```python
from build123d import *

# Parameters (mm, degrees)
F0_W     = 60
F0_H     = 40
F1_DEPTH = 70
F2_R     = 7.749318
F3_DEPTH = 15
F4_R     = 12.316216
F5_DEPTH = 15
F6_W     = 4.257482
F6_H     = 2.289564
F7_DEPTH = 5


with BuildPart() as f1:
    # F0 (on Top) → F1 (new body)
    with BuildSketch(Plane.XY):
        with Locations((-16.059712, 9.84915)):
            Rectangle(F0_W, F0_H)
    extrude(amount=F1_DEPTH)

    # F2 (on face) → F3 (join)
    with BuildSketch(Plane.XY.offset(70)):
        with Locations((-16.059712, 9.84915)):
            Circle(F2_R)
    extrude(amount=F3_DEPTH)

    # F4 (on face) → F5 (join)
    with BuildSketch(Plane.XY.offset(85)):
        with Locations((-16.059712, 9.84915)):
            Circle(F4_R)
    extrude(amount=F5_DEPTH)

    # F6 (on face) → F7 (join)
    with BuildSketch(Plane.XY.offset(100)):
        with Locations((-13.930971, 8.704368)):
            Rectangle(F6_W, F6_H)
    extrude(amount=F7_DEPTH)

    # F8 (on face) → F9 (revolve)
    with BuildSketch(Plane(origin=(0, 9.84915, 0), x_dir=(-1, 0, 0), z_dir=(0, 1, 0))):
        with BuildLine():
            Line((16.059712, 90.969634), (16.059712, 100))
            Line((16.059712, 100), (11.80223, 100))
            Line((11.80223, 100), (11.80223, 105))
            Line((11.80223, 105), (16.059712, 105))
            Line((16.059712, 105), (16.059712, 109.030366))
            ThreePointArc((16.059712, 109.030366), (2.458365, 103.762126), (-3.528251, 90.461321))
            Line((-3.528251, 90.461321), (16.059712, 90.969634))
        make_face()
    revolve(axis=Axis((-16.059712, 9.84915, 95.484817), (0, 0, -1)))


solid = f1.part
```
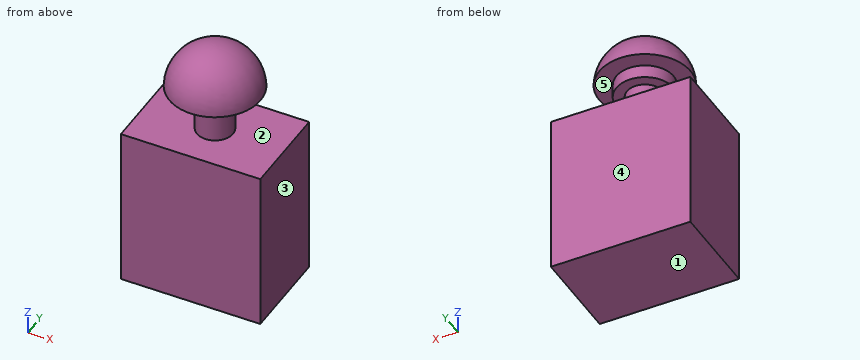
Source: CAD feature listing. Evaluate the final solid. Frame: model axes, mm. Face numbers are marked on the shaded views. A direction names the side the tool comes from. Coordinates: 2 decimals unless noted, no trailing zeros. Order: outer loops, then holes, each group sorted by start corner. A loop starts at its lowest first (then second) coordinate and runs counter-clockwise, first axis right, second up. Notation, with made-up numbers: M 49.5,42 L 84.5,42 A4 ccw 84.5,48 Z; hole C 22,2.25 d5. An arc over 180 degrees is marked long. Write each question's results on one line, items separated by ' | '. Start each with the question number.
1) Draft query along X for the marked faces 3, 4 and 5. Return one class per face: released by +X, released by -X, zero draft, split by the parting line, or undercut.
2) Contact query for flat-ended pins moving along their axis: pin 1 Ø5 at (x, y) = (-25.5, 10) entering from +Z; pin 2 Ø1.8 at (y, z) = (8.5, 102) entering from -X; pin 3 Ø1 at (x, y) = (-6, 2.5) entering from +Z. Output: stop coordinate, or through.
3) Section query A-A (x = -40). Return the cut outline in (y, z), plus the area to 3 significant figures.
4) Line query: line 1 (Z direction, x = 9.5, y = 11); line 2 (Z direction, x = -15, y = 19); line 3 (Z direction, x = -25, y = 7). Output: solid intervals per line, ascending. Write a range as from..to.
5) Access query for the marked faces 1 and 2. Directions: +Z, -Z, +X, -X, +Y, -Y. A direction counts if a zero-diameter tool reaches every point of the face in a straight line with its end or side. Return the directions, or none.
Answers:
1) face 3: released by +X | face 4: zero draft | face 5: undercut
2) pin 1: stops at z = 107.88 | pin 2: stops at x = -31.94 | pin 3: stops at z = 105.15
3) outline: M -10.15,0 L 29.85,0 L 29.85,70 L -10.15,70 Z | area: 2,800 mm^2
4) line 1: z = 0..70 | line 2: z = 0..70, 85..106.88 | line 3: z = 0..70, 85..106.79
5) face 1: -Z, +X, -X, +Y, -Y | face 2: none
